from build123d import *

# Parameters (mm, degrees)
CORTAR_EXTRUIR1_DEPTH = 21


with BuildPart() as part:
    # Croquis1 → Revolución2 (revolve)
    with BuildSketch(Plane.XY):
        Polygon((7.9375, 0), (7.9375, 20), (30.875, 20), (30.875, 16.35), (22.9375, 13.175), (22.9375, 6.825), (30.875, 3.65), (30.875, 0), align=None)
    revolve(axis=Axis((0, 0, 0), (0, 1, 0)))

    # Croquis2 → Cortar-Extruir1 (cut, through all)
    with BuildSketch(Plane(origin=(0, 20, 0), x_dir=(1, 0, 0), z_dir=(0, 1, 0))):
        with BuildLine():
            Line((-3.175, 11.1125), (-3.175, 7.274838916))
            ThreePointArc((-3.175, 7.274838916), (0, 7.9375), (3.175, 7.274838916))
            Line((3.175, 7.274838916), (3.175, 11.1125))
            Line((3.175, 11.1125), (-3.175, 11.1125))
        make_face()
    extrude(amount=-CORTAR_EXTRUIR1_DEPTH, mode=Mode.SUBTRACT)


solid = part.part
Geometry check sheet. Reference: the model listing, model coordinates, mm. A direction names the side the tool comes from. Coordinates: 2 decimals unless noted, no trailing zeros. Order: outer loops, then holes, each group sorted by start corner. A loop starts at its lowest first (then second) coordinate and runs counter-clockwise, first axis right, second up. Notation, with made-up numbers: M -13,-22 L 2,-22 A16 cw 2,0 Z; hole C 62,38.25 d8. An arc over 180 degrees is marked long. Use CSV: the item, a comma, the result in double quotes.
Item 1: Mould release check, pull along Y, two halves, no side actions. Record for faces 1 (the flat face through (3.175, 10, -9)), 2 (the flat face through (-6, 20, 6)), 3 (the conical face through (22.352, 6.626, -7.039)): pulls with the +Y half, pulls with the -Y half, needs draft (parallel to the pull), parting line crosses it, or undercut.
Returned:
face 1,"needs draft"
face 2,"pulls with the +Y half"
face 3,"undercut"
Item 2: Tool access check on faces 4 (the flat face through (6, 0, 6)), 5 (the flat face through (0, 10, -11.112)), 6 (the cylindrical face through (-2.99, 9.96, -22.74)). Record the directions out of +Z, -Z, +X, -X, +Y, -Y that give a thin tool (end or side, any length) a straight path to the whole face; none if there is none.
Returned:
face 4,"+Z, -Z, +X, -X, -Y"
face 5,"+Y, -Y"
face 6,"none"
Item 3: Gauge pin test, flat ends, axial feed: pin 1 Ø5 at (x, y) = (0, 12.5) entering from +Z; pin 2 Ø1.5 at (y, z) = (2.5, 18.5) entering from +X; pin 3 Ø18.5 at (x, z) = (0, 0) entering from +Y; pin 4 Ø5 at (x, y) = (-20.5, 2) entering from -Z. Record the tip position at first contact, or that the pin passes through.
Returned:
pin 1,"stops at z = 27.5"
pin 2,"stops at x = 25.26"
pin 3,"stops at y = 20"
pin 4,"stops at z = -25.09"
Item 4: Cross-section at D-D on y = 6. Record the cut outline in (x, z) (1 decimal), then the cut area to 3 significant figures.
Returned:
outline,"C 0,0 d50; hole M -3.2,-11.1 L 3.2,-11.1 L 3.2,-7.3 A7.9 ccw long -3.2,-7.3 Z"
area,"1,740 mm2"
Item 5: Cross-section at C-C on y = 10.5. Record the cut outline in (x, z) (1 decimal).
Returned:
outline,"C 0,0 d45.9; hole M -3.2,-11.1 L 3.2,-11.1 L 3.2,-7.3 A7.9 ccw long -3.2,-7.3 Z"
Item 6: Thickness scan on line 1 along X through (y, z) = (12, 0); line 2 along Z through (x, y) = (0, 14); line 3 along X through (y, z) = (13.5, 0). Record the ranges inside material, lowest first.
Returned:
line 1,"x = -22.94 to -7.94, 7.94 to 22.94"
line 2,"z = -25 to -11.11, 7.94 to 25"
line 3,"x = -23.75 to -7.94, 7.94 to 23.75"
